For this review, take the finished solid that the model builds, in its own axes (mm). A direction names the side the tool comes from. Round coordinates to 2 decimals unless told otherwise and drop trailing zeros. Loops run counter-clockwise (first coordinate to the right, second up) from the corner with the lowest first, then second, coordinate; pieces in that order, holes last. Notation, with made-up numbers: (-1, 71.5) -> (30, 71.5) arc R24 ccw to (30, 110.5) -> close; hole circle Ø10 at (54, 22.25). An arc over 180 degrees is marked (long way). Write each question's results on one line, items separated by ' | '.
```python
from build123d import *

# Parameters (mm, degrees)
SKETCH_1_R          = 2
EXTRUDE_1_DEPTH     = 5
EXTRUDE_2_DEPTH     = 15
SKETCH_5_W          = 10
SKETCH_5_H          = 7.614001554
CUT_EXTRUDE_2_DEPTH = 6
SKETCH_4_R          = 1.6
CUT_EXTRUDE_1_DEPTH = 40.982946782
FILLET_2_R          = 5
FILLET_3_R          = 2


with BuildPart() as part:
    # 草图1 → 凸台-拉伸1 (new body)
    with BuildSketch(Plane(origin=(0, 0, 0), x_dir=(1, 0, 0), z_dir=(0, 1, 0))):
        with BuildLine():
            ThreePointArc((20.794105787, -7.183673469), (0, 22), (-20.794105787, -7.183673469))
            ThreePointArc((-20.794105787, -7.183673469), (-22.340745823, -10.362966567), (-25.520038921, -8.816326531))
            ThreePointArc((-25.520038921, -8.816326531), (-26.229531343, -6.404036657), (-26.711538462, -3.936205408))
            ThreePointArc((-26.711538462, -3.936205408), (-30, 0), (-26.711538462, 3.936205408))
            ThreePointArc((-26.711538462, 3.936205408), (0, 27), (26.711538462, 3.936205408))
            ThreePointArc((26.711538462, 3.936205408), (30, 0), (26.711538462, -3.936205408))
            ThreePointArc((26.711538462, -3.936205408), (26.229531343, -6.404036657), (25.520038921, -8.816326531))
            ThreePointArc((25.520038921, -8.816326531), (22.340745823, -10.362966567), (20.794105787, -7.183673469))
        make_face()
        with Locations((-26, 0)):
            Circle(SKETCH_1_R, mode=Mode.SUBTRACT)
        with Locations((26, 0)):
            Circle(SKETCH_1_R, mode=Mode.SUBTRACT)
    extrude(amount=EXTRUDE_1_DEPTH)

    # 草图3 → 凸台-拉伸2 (add)
    with BuildSketch(Plane(origin=(0, 0, 0), x_dir=(1, 0, 0), z_dir=(0, 1, 0))):
        Polygon((-5, 33.807000777), (-9.982946782, 33.807000777), (-9.982946782, 22.896387671), (9.982946782, 22.896387671), (9.982946782, 33.807000777), (5, 33.807000777), (5, 26.192999223), (-5, 26.192999223), align=None)
    extrude(amount=EXTRUDE_2_DEPTH)

    # 草图5 → 切除-拉伸2 (cut, through all)
    with BuildSketch(Plane(origin=(0, 5, 0), x_dir=(1, 0, 0), z_dir=(0, 1, 0))):
        with Locations((0, 30)):
            Rectangle(SKETCH_5_W, SKETCH_5_H)
    extrude(amount=-CUT_EXTRUDE_2_DEPTH, mode=Mode.SUBTRACT)

    # 草图4 → 切除-拉伸1 (cut, through all)
    with BuildSketch(Plane.ZY.offset(9.982946782)):
        with Locations((-30, 4)):
            Circle(SKETCH_4_R)
        with Locations((-30, 11)):
            Circle(SKETCH_4_R)
    extrude(amount=-CUT_EXTRUDE_1_DEPTH, mode=Mode.SUBTRACT)

    # 圆角2
    fillet_2_edges = [part.edges().sort_by_distance(p)[0] for p in [
        (9.982946782, 2.5, -25.086665254),
        (-9.982946782, 2.5, -25.086665254),
    ]]
    fillet(fillet_2_edges, radius=FILLET_2_R)

    # 圆角3
    fillet_3_edges = [part.edges().sort_by_distance(p)[0] for p in [
        (-9.982946782, 10, -22.896387671),
        (9.982946782, 10, -22.896387671),
    ]]
    fillet(fillet_3_edges, radius=FILLET_3_R)


solid = part.part
```
1. To check wall thickness, follow probe 1 along Y at (x, z) = (-8.75, -30); probe 2 along X at (y, z) = (1.45, 0); probe 3 along X at (y, z) = (13.25, -28.5). State the ranges of each line that lie inside material, in increasing order.
Values found:
probe 1: y = 0 to 2.4, 5.6 to 9.4, 12.6 to 15 | probe 2: x = -30 to -28, -24 to -22, 22 to 24, 28 to 30 | probe 3: x = -9.98 to -5, 5 to 9.98
2. Tool access review of faces 1 (the face through (-9.983, 7, -29)), 2 (the face through (5, 8, -30)), 3 (the face through (0, 10, -22.896)), 4 (the face through (9.413, 10.07, -23.498)): name each direction out of +Z, -Z, +X, -X, +Y, -Y from which nothing blocks a thin tool from reaching the whole face with its end or side.
Values found:
face 1: -Z, -X, +Y | face 2: -Z, +Y, -Y | face 3: +Z, +X, -X, +Y | face 4: +Z, +X, +Y
3. Consider section A-A (z = -30). State the section outline as (x, y) points, plus the area to 3 significant figures.
Values found:
outline: (-9.98, 0) -> (-5, 0) -> (-5, 2.4) -> (-9.98, 2.4) -> close; (-9.98, 5.6) -> (-5, 5.6) -> (-5, 9.4) -> (-9.98, 9.4) -> close; (-9.98, 12.6) -> (-5, 12.6) -> (-5, 15) -> (-9.98, 15) -> close; (5, 0) -> (9.98, 0) -> (9.98, 2.4) -> (5, 2.4) -> close; (5, 5.6) -> (9.98, 5.6) -> (9.98, 9.4) -> (5, 9.4) -> close; (5, 12.6) -> (9.98, 12.6) -> (9.98, 15) -> (5, 15) -> close | area: 85.7 mm2
4. For pin 1 (2.5 mm diameter, centred on y = 10.5, z = -31, fed in from -X); pin 2 (3 mm diameter, centred on x = 10, z = -18, fed in from +Y); pin 3 (6 mm diameter, centred on y = 10, z = -29.5, fed in from +X), all flat-tipped, find the tip position at first contact; note any pin that passes through.
Values found:
pin 1: stops at x = -9.98 | pin 2: stops at y = 5 | pin 3: stops at x = 9.98
5. Consider section B-B (y = 4). State the section outline as (x, z) points, plus the area to 3 significant figures.
Values found:
outline: (-26.71, -3.94) arc R27 ccw to (-12.64, -23.86) arc R5 cw to (-9.98, -28.28) -> (-9.98, -28.4) -> (-5, -28.4) -> (-5, -26.19) -> (5, -26.19) -> (5, -28.4) -> (9.98, -28.4) -> (9.98, -28.28) arc R5 cw to (12.64, -23.86) arc R27 ccw to (26.71, -3.94) arc R4 ccw to (26.71, 3.94) arc R27 ccw to (25.52, 8.82) arc R2.5 ccw to (20.79, 7.18) arc R22 cw (long way) to (-20.79, 7.18) arc R2.5 ccw to (-25.52, 8.82) arc R27 ccw to (-26.71, 3.94) arc R4 ccw to start; (-9.98, -33.81) -> (-5, -33.81) -> (-5, -31.6) -> (-9.98, -31.6) -> close; (5, -33.81) -> (9.98, -33.81) -> (9.98, -31.6) -> (5, -31.6) -> close; hole circle Ø4 at (-26, 0); hole circle Ø4 at (26, 0) | area: 541 mm2
6. Draft analysis for pull direction X (two halves, no side actions). For faces 5 (the face through (0, 7, -26.193)), 6 (the face through (26.238, 2.465, 6.37)), 7 (the face through (4, 0, -22)), state which applies: released by +X, released by -X, zero draft, split by the parting line, or undercut.
Values found:
face 5: undercut | face 6: released by +X | face 7: zero draft
7. Consider section C-C (y = 7.25). State the section outline as (x, z) points, plus the area to 3 significant figures.
Values found:
outline: (-9.98, -33.81) -> (-5, -33.81) -> (-5, -26.19) -> (5, -26.19) -> (5, -33.81) -> (9.98, -33.81) -> (9.98, -24.9) arc R2 ccw to (7.98, -22.9) -> (-7.98, -22.9) arc R2 ccw to (-9.98, -24.9) -> close | area: 140 mm2
8. Consider section D-D (z = 8). State the section outline as (x, y) points, plus the area to 3 significant figures.
Values found:
outline: (-25.79, 0) -> (-20.66, 0) -> (-20.66, 5) -> (-25.79, 5) -> close; (20.66, 0) -> (25.79, 0) -> (25.79, 5) -> (20.66, 5) -> close | area: 51.3 mm2
